Geometry check sheet. Reference: the model listing, model coordinates, mm. Face numbers are marked on the shaded views. A direction names the side the tool comes from. Give positions to 0.01 mm unless a question says otherwise; leave off trailing zeros. Loops run counter-clockwise (first coordinate to the right, second up) from the corner with the lowest first, then second, coordinate; pieces in that order, holes last. Notation, with made-up numbers: (14, -20.75) - (52, -20.75) arc R30 ccw to (52, 17.25) - close; hole circle Ø2 at (-13, 31). An arc over 180 degrees is marked (long way). Use a Markdown table: item, result. Add a question column.
1. Set-up check for the marked faces 1, 2, 3 and 4: record each of +Z, -Z, +X, -X, +Y, -Y from which the full face is reachable in a straight line by a thin tool's end or side.
2. Material ranges on L1, parallel to Z at x = -13.5, y = -17; L2, parallel to X at y = -4.75, z = 2; L3, parallel to Z at x = 13, y = -23.5, recorded low to high.
3. Cross-section at B-B on z = -7.5. Enter the section's corners in (x, y), and give its area (3 significant figures).
4. Depth check by flat-ended pin: P1, Ø1, axis at y = -7.5, z = 13, coming from the -X side; P2, Ø1, axis at y = -7, z = 15, coming from the +X side; P3, Ø12, axis at y = -20.5, z = 7, coming from the +X side. Enter the tip coordinate at first touch or a pass-through.
5. Cross-section at C-C on y = -8.75. Enter the section's corners in (x, z), and give its area (3 significant figures).
6. Cross-section at A-A on y = -12.7. Enter the section's corners in (x, z), and give its area (3 significant figures).
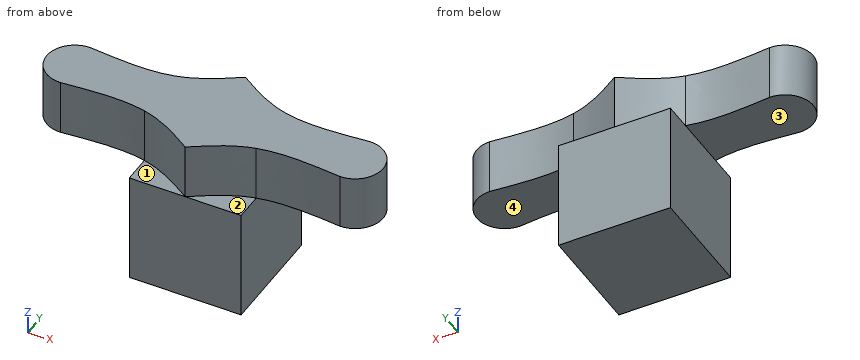
from build123d import *

# Parameters (mm, degrees)
F0_W     = 25.4
F0_H     = 38.1
F1_DEPTH = 25.4
F2_W     = 19.05
F2_H     = 12.7
F3_DEPTH = 12.7
F5_DEPTH = 12.7
F7_DEPTH = 12.7


with BuildPart() as f1:
    # F0 (on Front) → F1 (new body)
    with BuildSketch(Plane.XZ):
        with Locations((1.1045151994, 7.9051328331)):
            Rectangle(F0_W, F0_H)
    extrude(amount=F1_DEPTH)

    # F2 (on face) → F3 (join)
    with BuildSketch(Plane.XY.offset(26.9551328331)):
        with Locations((-21.1204848006, -12.7)):
            Rectangle(F2_W, F2_H)
        Polygon((13.8045151994, -6.35), (13.8045151994, -19.05), (32.860204035, -19.05), (32.8545151994, -6.35), align=None)
    extrude(amount=-F3_DEPTH)

    # F4 (on face) → F5 (cut)
    with BuildSketch(Plane.XY.offset(26.9551328331)):
        with BuildLine():
            Line((-11.5954848006, -19.05), (-11.5954848006, -25.4))
            Line((-11.5954848006, -25.4), (1.1045151994, -25.4))
            add(Edge.make_bspline(
                [(1.1045151994, -25.4), (-2.8394977605, -22.7929764945), (-6.7835107203, -20.1859529889), (-11.5954848006, -19.05)],
                knots=[0, 0, 0, 0, 0.4633292966, 0.4633292966, 0.4633292966, 0.4633292966], degree=3))
        make_face()
        with BuildLine():
            add(Edge.make_bspline(
                [(1.1045151994, -25.4), (5.0483617358, -22.7930157817), (8.9922082723, -20.1860315634), (13.8045151994, -19.05)],
                knots=[0, 0, 0, 0, 0.4632921748, 0.4632921748, 0.4632921748, 0.4632921748], degree=3))
            Line((1.1045151994, -25.4), (13.8045151994, -25.4))
            Line((13.8045151994, -25.4), (13.8045151994, -19.05))
        make_face()
        with BuildLine():
            add(Edge.make_bspline(
                [(1.1045151994, 0), (5.0485281592, -2.6070235055), (8.992541119, -5.2140470111), (13.8045151994, -6.35)],
                knots=[0, 0, 0, 0, 0.4633292966, 0.4633292966, 0.4633292966, 0.4633292966], degree=3))
            Line((13.8045151994, -6.35), (13.8045151994, 0))
            Line((13.8045151994, 0), (1.1045151994, 0))
        make_face()
        with BuildLine():
            Line((-11.5954848006, 0), (-11.5954848006, -6.35))
            add(Edge.make_bspline(
                [(1.1045151994, 0), (-2.8394977605, -2.6070235055), (-6.7835107203, -5.2140470111), (-11.5954848006, -6.35)],
                knots=[0, 0, 0, 0, 0.4633292966, 0.4633292966, 0.4633292966, 0.4633292966], degree=3))
            Line((1.1045151994, 0), (-11.5954848006, 0))
        make_face()
        with BuildLine():
            add(Edge.make_bspline(
                [(13.8045151994, -19.05), (19.3794049248, -17.7339470577), (26.1198044799, -18.3919735289), (32.860204035, -19.05)],
                knots=[0.4632921748, 0.4632921748, 0.4632921748, 0.4632921748, 1, 1, 1, 1], degree=3))
            Line((13.8045151994, -19.05), (32.860204035, -19.05))
        make_face()
        with BuildLine():
            add(Edge.make_bspline(
                [(13.8045151994, -6.35), (19.3781871724, -7.6657654699), (26.1163511859, -7.007882735), (32.8545151994, -6.35)],
                knots=[0.4633292966, 0.4633292966, 0.4633292966, 0.4633292966, 1, 1, 1, 1], degree=3))
            Line((32.8545151994, -6.35), (13.8045151994, -6.35))
        make_face()
        with BuildLine():
            Line((-11.5954848006, -6.35), (-30.6454848006, -6.35))
            add(Edge.make_bspline(
                [(-11.5954848006, -6.35), (-17.1691567737, -7.6657654699), (-23.9073207872, -7.007882735), (-30.6454848006, -6.35)],
                knots=[0.4633292966, 0.4633292966, 0.4633292966, 0.4633292966, 1, 1, 1, 1], degree=3))
        make_face()
        with BuildLine():
            Line((-30.6454848006, -19.05), (-11.5954848006, -19.05))
            add(Edge.make_bspline(
                [(-11.5954848006, -19.05), (-17.1691567737, -17.7342345301), (-23.9073207872, -18.392117265), (-30.6454848006, -19.05)],
                knots=[0.4633292966, 0.4633292966, 0.4633292966, 0.4633292966, 1, 1, 1, 1], degree=3))
        make_face()
    extrude(amount=-F5_DEPTH, mode=Mode.SUBTRACT)

    # F6 (on face) → F7 (join)
    with BuildSketch(Plane.XY.offset(26.9551328331)):
        with BuildLine():
            ThreePointArc((32.860204035, -19.05), (39.2073596172, -12.6971555822), (32.8545151994, -6.35))
            Line((32.8545151994, -6.35), (32.860204035, -19.05))
        make_face()
        with BuildLine():
            Line((-30.6454848006, -19.05), (-30.6454848006, -6.35))
            ThreePointArc((-30.6454848006, -6.35), (-37.1683022833, -12.7), (-30.6454848006, -19.05))
        make_face()
    extrude(amount=-F7_DEPTH)


solid = f1.part
Values found:
| question | item | result |
|---|---|---|
| 1 | face 1 | +Z, -X, -Y |
| 1 | face 2 | +Z, +X, -Y |
| 1 | face 3 | -Z, -X, +Y, -Y |
| 1 | face 4 | -Z, +X, +Y, -Y |
| 2 | L1 | z = 14.26 to 26.96 |
| 2 | L2 | x = -11.6 to 13.8 |
| 2 | L3 | z = -11.14 to 14.26 |
| 3 | outline | (-11.6, -25.4) - (13.8, -25.4) - (13.8, 0) - (-11.6, 0) - close |
| 3 | area | 645 mm2 |
| 4 | P1 | stops at x = -11.6 |
| 4 | P2 | stops at x = 36.5 |
| 4 | P3 | stops at x = 13.8 |
| 5 | outline | (-35.79, 14.26) - (-11.6, 14.26) - (-11.6, -11.14) - (13.8, -11.14) - (13.8, 14.26) - (37.83, 14.26) - (37.83, 26.96) - (-35.79, 26.96) - close |
| 5 | area | 1,580 mm2 |
| 6 | outline | (-37.17, 14.26) - (-11.6, 14.26) - (-11.6, -11.14) - (13.8, -11.14) - (13.8, 14.26) - (39.21, 14.26) - (39.21, 26.96) - (-37.17, 26.96) - close |
| 6 | area | 1,620 mm2 |
